```python
from build123d import *

# Parameters (mm, degrees)
SKETCH3_R           = 14.125
SKETCH3_R_2         = 6
BOSS_EXTRUDE1_DEPTH = 5
BOSS_EXTRUDE2_START = -5
SKETCH4_R           = 6
SKETCH4_R_2         = 5
BOSS_EXTRUDE2_DEPTH = 1
SKETCH5_R           = 1.5
CUT_EXTRUDE1_DEPTH  = 10
CHAMFER1_SIZE       = 0.5


with BuildPart() as part:
    # Sketch3 → Boss-Extrude1 (new body)
    with BuildSketch(Plane.YZ):
        with Locations(Location((0, 0, 0), (0, 0, 270))):
            Circle(SKETCH3_R)
        with Locations(Location((0, 0, 0), (0, 0, 270))):
            Circle(SKETCH3_R_2, mode=Mode.SUBTRACT)
    extrude(amount=BOSS_EXTRUDE1_DEPTH)

    # Sketch4 → Boss-Extrude2 (add)
    with BuildSketch(Plane.YZ.offset(5).offset(BOSS_EXTRUDE2_START)):
        with Locations(Location((0, 0, 0), (0, 0, 270))):
            Circle(SKETCH4_R)
        with Locations(Location((0, 0, 0), (0, 0, 270))):
            Circle(SKETCH4_R_2, mode=Mode.SUBTRACT)
    extrude(amount=BOSS_EXTRUDE2_DEPTH)

    # Sketch5 → Cut-Extrude1 (cut)
    with BuildSketch(Plane(origin=(5, 0, 0), x_dir=(0, 0, -1), z_dir=(1, 0, 0))):
        with Locations((0, 10)):
            Circle(SKETCH5_R)
        with Locations((8.660254038, -5)):
            Circle(SKETCH5_R)
        with Locations((-8.660254038, -5)):
            Circle(SKETCH5_R)
    extrude(amount=-CUT_EXTRUDE1_DEPTH, mode=Mode.SUBTRACT)

    # Chamfer1
    chamfer1_edges = [part.edges().sort_by_distance(p)[0] for p in [
        (5, 0, 6),
    ]]
    chamfer(chamfer1_edges, length=CHAMFER1_SIZE)


solid = part.part
```
CAD build for the part. Positions are in the model's coordinates, mm. A direction names the side the tool comes from. Give positions to 0.01 mm unless a question says otherwise; leave off trailing zeros. Write each loop counter-clockwise with the first axis right and the second up, starting at its lowest first coordinate (ties: lowest second). Pieces come first, ordered by that corner, then holes. Notation, with made-up numbers: (2.25, 8.25) -> (18.25, 8.25) arc R18 cw to (18.25, 13.25) -> close; hole circle Ø3 at (85.5, 1.25). An arc over 180 degrees is marked (long way). Write each question's results on one line, items separated by ' | '.
1. Cut at C-C, the plane z = 8. Write the cut outline in (x, y), then the cut area to 3 significant figures.
Geometry check:
outline: (0, -11.64) -> (5, -11.64) -> (5, -6.35) -> (0, -6.35) -> close; (0, -3.65) -> (5, -3.65) -> (5, 11.64) -> (0, 11.64) -> close | area: 103 mm²
2. Two-plate mould, pull along Y, no slides. Class faces 1 (the flat face through (0, 0, -6)), 2 (the cylindrical face through (2.54, -3.74, 7.85)), 3 (the cylindrical face through (2.46, -5.41, -13.05)): pulls with the +Y half, pulls with the -Y half, needs draft (parallel to the pull), parting line crosses it, or undercut.
Geometry check:
face 1: needs draft | face 2: undercut | face 3: parting line crosses it
3. Cut at B-B, the plane y = 0. Write the cut outline in (x, z) (3 decimals), then the cut area to 3 significant figures.
Geometry check:
outline: (0, -14.125) -> (5, -14.125) -> (5, -6.5) -> (4.5, -6) -> (1, -6) -> (1, -5) -> (0, -5) -> close; (0, 5) -> (1, 5) -> (1, 6) -> (4.5, 6) -> (5, 6.5) -> (5, 14.125) -> (0, 14.125) -> close | area: 83.0 mm²
4. Drop flat-ended pins along their axis: P1, Ø9, axis at y = 0, z = 0, coming from the +X side; P2, Ø11, axis at y = 0, z = 0, coming from the +X side. Give the stop position or say it passes through.
Geometry check:
P1: through | P2: x = 1
5. Cut at A-A, the plane z = 0. Write the cut outline in (x, y) (3 decimals).
Geometry check:
outline: (0, -14.125) -> (5, -14.125) -> (5, -6.5) -> (4.5, -6) -> (1, -6) -> (1, -5) -> (0, -5) -> close; (0, 5) -> (1, 5) -> (1, 6) -> (4.5, 6) -> (5, 6.5) -> (5, 8.5) -> (0, 8.5) -> close; (0, 11.5) -> (5, 11.5) -> (5, 14.125) -> (0, 14.125) -> close
6. Which spindle directions (+Z, -Z, +X, -X, +Y, -Y) get a long thin tool onto all of the face, cutting with end or side? Do faces 4 (the flat face through (5, -3, -6)), 5 (the cylindrical face through (2.726, 1.802, -5.723)). Say none if no direction does.
Geometry check:
face 4: +Z, -Z, +X, +Y, -Y | face 5: +X
7. Wall check: probe 1 along Y at (x, z) = (2.3, 0) (3 decimals); probe 2 along Y at (x, z) = (3.9, 0.5); probe 3 along Y at (x, z) = (3.65, -9.25). Give the ranges that are in metal, low to high. Write a range as [from, to].
Geometry check:
probe 1: [-14.125, -6], [6, 8.5], [11.5, 14.125] | probe 2: [-14.12, -5.98], [5.98, 8.59], [11.41, 14.12] | probe 3: [-10.67, -6.38], [-3.62, 10.67]
8. Cut at D-D, the plane y = 10. Write the cut outline in (x, z), then the cut area to 3 significant figures.
Geometry check:
outline: (0, -9.98) -> (5, -9.98) -> (5, -1.5) -> (0, -1.5) -> close; (0, 1.5) -> (5, 1.5) -> (5, 9.98) -> (0, 9.98) -> close | area: 84.8 mm²
